from build123d import *

# Parameters (mm, degrees)
SKETCH1_R               = 4.5
BOSS_EXTRUDE1_DEPTH     = 19.5
SKETCH2_R               = 7
BOSS_EXTRUDE2_DEPTH     = 2
CUT_EXTRUDE1_DEPTH      = 22.868927729
CUT_EXTRUDE1_DEPTH_BACK = 22.868927729
SKETCH3_R               = 1.5


with BuildPart() as part:
    # Sketch1 → Boss-Extrude1 (new body)
    with BuildSketch(Plane(origin=(0, 0, 0), x_dir=(0, 0, -1), z_dir=(1, 0, 0))):
        Circle(SKETCH1_R)
    extrude(amount=BOSS_EXTRUDE1_DEPTH)

    # Sketch2 → Boss-Extrude2 (add)
    with BuildSketch(Plane.ZY):
        Circle(SKETCH2_R)
    extrude(amount=-BOSS_EXTRUDE2_DEPTH)

    # Sketch3 → Cut-Extrude1 (cut, two sides: drawn at the far end of the back side and taken through both)
    with BuildSketch(Plane(origin=(0, 0, 0), x_dir=(1, 0, 0), z_dir=(0, 1, 0)).offset(-CUT_EXTRUDE1_DEPTH_BACK)):
        with Locations(Location((15, 0, 0), (0, 0, 270))):
            Circle(SKETCH3_R)
    extrude(amount=CUT_EXTRUDE1_DEPTH + CUT_EXTRUDE1_DEPTH_BACK, mode=Mode.SUBTRACT)


solid = part.part
Geometry check sheet. Reference: the model listing, model coordinates, mm. A direction names the side the tool comes from. Coordinates: 2 decimals unless noted, no trailing zeros. Order: outer loops, then holes, each group sorted by start corner. A loop starts at its lowest first (then second) coordinate and runs counter-clockwise, first axis right, second up. Notation, with made-up numbers: (-29, -31) - (3, -31) arc R12 ccw to (3, -18) - close; hole circle Ø2 at (-32, 67.5). An arc over 180 degrees is marked (long way). One line per item, written item: value.
(1) Sectioned sample at D-D (z = -4). Enter the section's corners in (x, y).
Data:
outline: (0, -5.74) - (2, -5.74) - (2, -2.06) - (19.5, -2.06) - (19.5, 2.06) - (2, 2.06) - (2, 5.74) - (0, 5.74) - close
(2) Thickness scan on probe 1 along X at (y, z) = (1.75, 0); probe 2 along Z at (x, y) = (15, 1); probe 3 along Z at (x, y) = (15, 2). Record the ranges inside material, lowest first. Write a range as from..to.
Data:
probe 1: x = 0..13.5, 16.5..19.5
probe 2: z = -4.39..-1.5, 1.5..4.39
probe 3: z = -4.03..-1.5, 1.5..4.03
(3) Release check for a two-part mould opening along Z. For faces 1 (the face through (10.628, 1.352, -4.292)), 2 (the face through (19.5, 0, 0)), 3 (the face through (16.265, -0.063, 0.806)) record: +Z half, -Z half, draft (parallel to the pull), parting line (faces both ways), or undercut.
Data:
face 1: parting line
face 2: draft
face 3: undercut
(4) Sectioned sample at A-A (z = 0). Enter the section's corners in (x, y), and give its area (4 significant figures).
Data:
outline: (0, -7) - (2, -7) - (2, -4.5) - (13.5, -4.5) - (13.5, 4.5) - (2, 4.5) - (2, 7) - (0, 7) - close; (16.5, -4.5) - (19.5, -4.5) - (19.5, 4.5) - (16.5, 4.5) - close
area: 158.5 mm^2
(5) Depth check by flat-ended pin: pin 1 Ø1 at (x, z) = (5.5, 0.5) entering from +Y; pin 2 Ø4 at (x, z) = (3.5, 2.5) entering from -Y; pin 3 Ø3 at (x, y) = (6, 1) entering from +Z. Enter the tip coordinate at first touch or a pass-through.
Data:
pin 1: stops at y = 4.5
pin 2: stops at y = -6.9
pin 3: stops at z = 4.5
(6) Access from +Z, -Z, +X, -X, +Y, -Y to the whole of each face (thin tool, end or side, straight path). Record for faces 4 (the face through (0, 0, 0)), 5 (the face through (2, -5, 0)).
Data:
face 4: +Z, -Z, -X, +Y, -Y
face 5: +X
(7) Sectioned sample at B-B (y = 0). Enter the section's corners in (x, z), and give its area (3 significant figures).
Data:
outline: (0, -7) - (2, -7) - (2, -4.5) - (19.5, -4.5) - (19.5, 4.5) - (2, 4.5) - (2, 7) - (0, 7) - close; hole circle Ø3 at (15, 0)
area: 178 mm^2
(8) Sectioned sample at C-C (x = 14.5). Enter the section's corners in (y, z).
Data:
outline: (-4.27, -1.41) arc R4.5 ccw to (4.27, -1.41) - close; (-4.27, 1.41) - (4.27, 1.41) arc R4.5 ccw to start
